Could you check a few things on this drawing? It's one solid part, dimensions in mm from its lowest x, y, z. A direction names the side the tool comes from. Give positions to 0.01 mm unless a question says otherwise; leave off trailing zeros. Loops run counter-clockwise (first coordinate to the right, second up) from the corner with the lowest first, then second, coordinate; pieces in that order, holes last.
1. Imagine slicing it at B-B (x = 57). List the corners of the cut face in (y, z) for me, plus the area to 3 significant figures.
2. For the marked faces 4 and 5, which set-ups out of +Z, -Z, +X, -X, +Y, -Y let a thin tool reach every point of the face, with its end or its side?
3. For P1, Ø3.5, axis at y = 34.5, z = 2, coming from the +X side; P2, Ø1.5, axis at y = 39, z = 21, coming from the +X side; P3, Ø4, axis at x = 57, z = 40.32, coming from the +Y side, each with a flat end and sliding along its axis, tell me the tip position at first contact or that it passes through.
4. Thinking about a two-plate mould opening in Y: for the marked faces 1, 2 and 3, which applies, +Y half, -Y half, draft (parallel to the pull), parting line (faces both ways), or undercut?
5. Imagine slicing it at A-A (x = 32.5). List the corners of the cut face in (y, z) for me.
6. I need wall thicknesses on line 1 along Y through (x, z) = (34.5, 16); line 2 along Z through (x, y) = (18, 17); line 3 along X through (y, z) = (45, 21). Which ranges of each line are inside material? Lowest first, please.
7. Imagine slicing it at D-D (x = 48). List the corners of the cut face in (y, z) for me.
8. Imagine slicing it at C-C (y = 31). List the corners of the cut face in (x, z) for me.
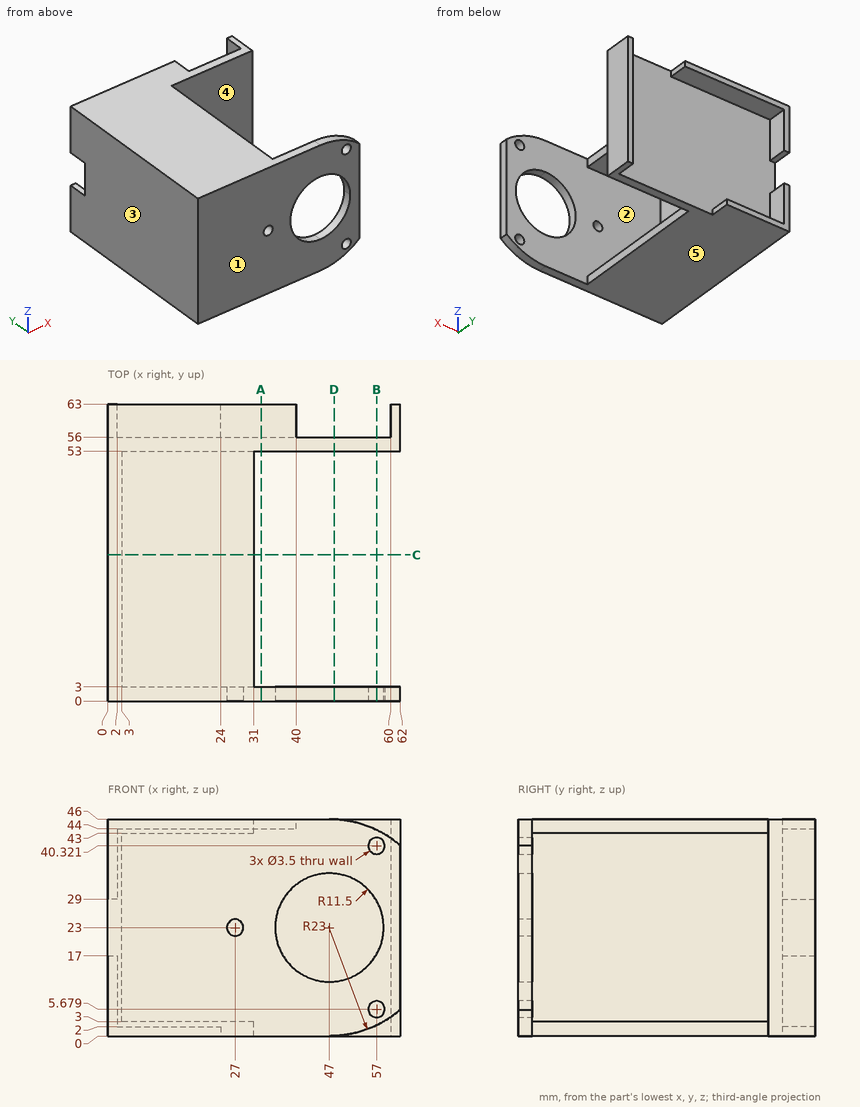
Derived:
1. outline: (0, 2.29) - (3, 2.29) - (3, 3.93) - (0, 3.93) - close; (0, 7.43) - (3, 7.43) - (3, 17.32) - (0, 17.32) - close; (0, 28.68) - (3, 28.68) - (3, 38.57) - (0, 38.57) - close; (0, 42.07) - (3, 42.07) - (3, 43.71) - (0, 43.71) - close; (53, 0) - (56, 0) - (56, 46) - (53, 46) - close
1. area: 207 mm2
2. face 4: +X
2. face 5: -Z, +X, -X, +Y, -Y
3. P1: stops at x = 31
3. P2: stops at x = 3
3. P3: stops at y = 56
4. face 1: -Y half
4. face 2: undercut
4. face 3: draft
5. outline: (0, 0) - (3, 0) - (3, 46) - (0, 46) - close; (53, 0) - (56, 0) - (56, 44) - (63, 44) - (63, 46) - (53, 46) - close
6. line 1: y = 0 to 3, 53 to 56
6. line 2: z = 0 to 3, 43 to 46
6. line 3: x = 0 to 3
7. outline: (0, 0.02) - (3, 0.02) - (3, 11.54) - (0, 11.54) - close; (0, 34.46) - (3, 34.46) - (3, 45.98) - (0, 45.98) - close; (53, 0) - (56, 0) - (56, 46) - (53, 46) - close
8. outline: (0, 0) - (31, 0) - (31, 3) - (3, 3) - (3, 43) - (31, 43) - (31, 46) - (0, 46) - close
